```python
from build123d import *

# Parameters (mm, degrees)
SKETCH_R     = 2.55
PAD_DEPTH    = 2
PAD001_DEPTH = 10.5
PAD002_DEPTH = 2


with BuildPart() as part:
    # Sketch → Pad (new body)
    with BuildSketch(Plane.XZ):
        with BuildLine():
            Line((-22.193171, 20), (-14.990659, 3.994417))
            Line((-14.990659, 3.994417), (-20.462188, 1.532229))
            ThreePointArc((-20.462188, 1.532229), (-23.866395, -5.198432), (-18, -9.9393))
            Line((-18, -9.9393), (18, -9.9393))
            ThreePointArc((18, -9.9393), (23.866395, -5.198432), (20.462188, 1.532229))
            Line((14.990659, 3.994417), (20.462188, 1.532229))
            Line((22.193171, 20), (14.990659, 3.994417))
            ThreePointArc((22.193171, 20), (16.710243, 23), (11.227315, 20))
            Line((11.227315, 20), (2.227315, 0))
            Line((-2.227315, 0), (2.227315, 0))
            Line((-11.227315, 20), (-2.227315, 0))
            ThreePointArc((-11.227315, 20), (-16.710243, 23), (-22.193171, 20))
        make_face()
        with Locations((-18, -3.9393)):
            Circle(SKETCH_R, mode=Mode.SUBTRACT)
        with Locations((18, -3.9393)):
            Circle(SKETCH_R, mode=Mode.SUBTRACT)
    extrude(amount=PAD_DEPTH)

    # Sketch001 (on Face16 of Pad) → Pad001 (join)
    with BuildSketch(Plane.XZ.offset(2)):
        Polygon((-20, 20), (-11, 0), (-13.193171, 0), (-22.193171, 20), align=None)
        Polygon((20, 20), (11, 0), (13.193171, 0), (22.193171, 20), align=None)
    extrude(amount=PAD001_DEPTH)

    # Sketch002 (on Face25 of Pad001) → Pad002 (join)
    with BuildSketch(Plane.XZ.offset(12.5)):
        with BuildLine():
            Line((-22.193171, 20), (-13.193171, 0))
            ThreePointArc((-13.193171, 0), (-9.355122, -2), (-5.517072, 0))
            Line((-14.517072, 20), (-5.517072, 0))
            ThreePointArc((-14.517072, 20), (-18.355122, 22), (-22.193171, 20))
        make_face()
        with BuildLine():
            Line((22.193171, 20), (13.193171, 0))
            ThreePointArc((5.517072, 0), (9.355122, -2), (13.193171, 0))
            Line((14.517072, 20), (5.517072, 0))
            ThreePointArc((22.193171, 20), (18.355122, 22), (14.517072, 20))
        make_face()
    extrude(amount=PAD002_DEPTH)


solid = part.part
```
Verification items for the finished model (mm, model axes). A direction names the side the tool comes from. Give positions to 0.01 mm unless a question says otherwise; leave off trailing zeros. Order: outer loops, then holes, each group sorted by start corner. A loop starts at its lowest first (then second) coordinate and runs counter-clockwise, first axis right, second up. Notation, with made-up numbers: M 77.5,14.5 L 128.5,14.5 A31 ccw 128.5,47.5 Z; hole C 37.25,-29.75 d9. An arc over 180 degrees is marked long. Return JSON: item names as keys, results as strings. Group by question number.
1) Scan lines: line 1 (X direction, y = -0.5, z = -4); line 2 (Y direction, x = -15, z = 20); line 3 (Z direction, x = -18, y = -0.95). Record each from-to range of solid material in increasing order.
2) Access from +Z, -Z, +X, -X, +Y, -Y to the whole of each face (thin tool, end or side, straight path). Record for faces 4 (the face through (-17.69, -0.99, 2.78)), 5 (the face through (21, -7, 20)), 6 (the face through (10.08, -13.49, 10.14)), 7 (the face through (0, -1, 0)).
3) Section check A-A on y = -4. Record the cut outline in (x, z).
4) Section check B-B on x = -10. Record the cut outline in (y, z), and give its area (3 significant figures).
5) Section check C-C on z = -3. Record the cut outline in (x, y).
6) Mould release check, pull along Z, two halves, no side actions. Record for faces 1 (the face through (0, 0, -1)), 2 (the face through (17.69, -0.99, 2.78)), 3 (the face through (17.63, -8.16, 9.86)): pulls with the +Z half, pulls with the -Z half, needs draft (parallel to the pull), parting line crosses it, or undercut.
7) Section check D-D on z = 5.5. Record the cut outline in (x, y) (3 decimals).
8) Go/stop test with flat-tipped pins: pin 1 Ø1.1 at (x, y) = (-21, -6.5) entering from +Z; pin 2 Ø2 at (y, z) = (-10.5, 5.5) entering from +X; pin 3 Ø1.8 at (x, y) = (12, -6) entering from -Z; pin 4 Ø3 at (x, z) = (-18, -3.94) entering from -Y. Record where each tip stops, or that it passes through.
Answer block:
{
 "1": {"line 1": "x = -24 to -20.55, -15.45 to 15.45, 20.55 to 24", "line 2": "y = -14.5 to -12.5, -2 to 0", "line 3": "z = -9.94 to -6.49, -1.39 to 2.64, 10.68 to 22.87"},
 "2": {"face 4": "-X, +Y, -Y", "face 5": "+Z, +X, -X", "face 6": "+Z, -Y", "face 7": "+Z, +Y, -Y"},
 "3": {"outline": "M -22.19,20 L -13.19,0 L -11,0 L -20,20 Z; M 11,0 L 13.19,0 L 22.19,20 L 20,20 Z"},
 "4": {"outline": "M -14.5,-1.96 L -12.5,-1.96 L -12.5,9.96 L -14.5,9.96 Z; M -2,-9.94 L 0,-9.94 L 0,17.27 L -2,17.27 Z", "area": "78.3 mm^2"},
 "5": {"outline": "M -23.93,-2 L -20.37,-2 L -20.37,0 L -23.93,0 Z; M -15.63,-2 L 15.63,-2 L 15.63,0 L -15.63,0 Z; M 20.37,-2 L 23.93,-2 L 23.93,0 L 20.37,0 Z"},
 "6": {"face 1": "needs draft", "face 2": "undercut", "face 3": "pulls with the -Z half"},
 "7": {"outline": "M -15.668,-14.5 L -7.992,-14.5 L -7.992,-12.5 L -13.475,-12.5 L -13.475,-2 L -4.702,-2 L -4.702,0 L -15.668,0 Z; M 4.702,-2 L 13.475,-2 L 13.475,-12.5 L 7.992,-12.5 L 7.992,-14.5 L 15.668,-14.5 L 15.668,0 L 4.702,0 Z"},
 "8": {"pin 1": "stops at z = 20", "pin 2": "stops at x = 16.12", "pin 3": "stops at z = 0", "pin 4": "passes through"}
}
